```python
from build123d import *

# Parameters (mm, degrees)
BASE_EXTRUDE_DEPTH = 5.55625
SKETCH4_R          = 3.175
I_D_DEPTH          = 6.55625
SKETCH5_OUTSIDE_W  = 106.392
SKETCH5_OUTSIDE_H  = 104.672
SKETCH5_OUTSIDE_R  = 5.55625
CUT_EXTRUDE3_DEPTH = 25.4
CUT_EXTRUDE3_TAPER = 60
SKETCH6_OUTSIDE_W  = 53.046
SKETCH6_OUTSIDE_H  = 51.326
SKETCH6_OUTSIDE_R  = 5.55625
CUT_EXTRUDE4_DEPTH = 10
CUT_EXTRUDE4_TAPER = 60


with BuildPart() as part:
    # Sketch2 → Base-Extrude (new body)
    with BuildSketch(Plane.XY):
        Polygon((3.207902433, -5.55625), (6.415804866, 0), (3.207902433, 5.55625), (-3.207902433, 5.55625), (-6.415804866, 0), (-3.207902433, -5.55625), align=None)
    extrude(amount=-BASE_EXTRUDE_DEPTH)

    # Sketch4 → I.D. (cut, through all)
    with BuildSketch(Plane.XY):
        Circle(SKETCH4_R)
    extrude(amount=-I_D_DEPTH, mode=Mode.SUBTRACT)

    # Sketch5 outside → Cut-Extrude3 (cut)
    with BuildSketch(Plane(origin=(0, 0, -5.55625), x_dir=(-1, 0, 0), z_dir=(0, 0, -1))):
        Rectangle(SKETCH5_OUTSIDE_W, SKETCH5_OUTSIDE_H)
        Circle(SKETCH5_OUTSIDE_R, mode=Mode.SUBTRACT)
    extrude(amount=-CUT_EXTRUDE3_DEPTH, taper=CUT_EXTRUDE3_TAPER, mode=Mode.SUBTRACT)

    # Sketch6 outside → Cut-Extrude4 (cut)
    with BuildSketch(Plane.XY):
        Rectangle(SKETCH6_OUTSIDE_W, SKETCH6_OUTSIDE_H)
        Circle(SKETCH6_OUTSIDE_R, mode=Mode.SUBTRACT)
    extrude(amount=-CUT_EXTRUDE4_DEPTH, taper=CUT_EXTRUDE4_TAPER, mode=Mode.SUBTRACT)


solid = part.part
```
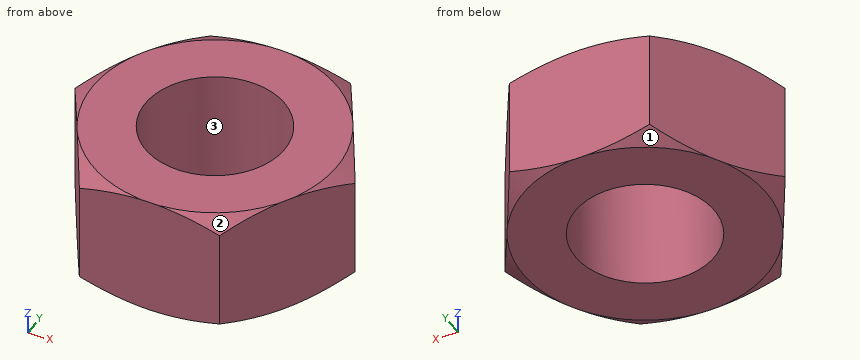
Geometry: final body of the model. Coordinates: model frame, mm. Face numbers are marked on the shaded views. Coordinates: 2 decimals unless noted, no trailing zeros. Loops run counter-clockwise (first coordinate to the right, second up) from the corner with the lowest first, then second, coordinate; pieces in that order, holes last. Notation, with made-up numbers: (-4, 69.5) -> (33, 69.5) arc R33 ccw to (33, 98.5) -> close; hole circle Ø10 at (28.25, -33). An arc over 180 degrees is marked (long way). Use a Markdown table: item, result. Add a question column.
(1) Line query: line 1 along Y through (x, z) = (0, -4.3) (3 decimals); line 2 along X through (y, z) = (-1.75, -2.55); line 3 along Y through (x, z) = (2.5, -4.2). Output: solid intervals per line, ascending.
(2) Mould query, pull axis X, two halves, no side actions, for the marked faces 1, 2 and 3. Classes: pulls with the +X half, pulls with the -X half, needs draft (parallel to the pull), parting line crosses it, or undercut.
(3) Section query A-A, the plane z = -1.45. Return loops of the section in (x, y) (3 decimals), plus the area to 3 significant figures.
(4) Pin query (flat end, axial travel): pin 1 Ø1.5 at (y, z) = (-1, -5) entering from +X; pin 2 Ø5.5 at (x, y) = (0, 0) entering from +Z. Return the tip coordinate at first contact, or that it passes through.
Answer:
| question | item | result |
|---|---|---|
| 1 | line 1 | y = -5.556 to -3.175, 3.175 to 5.556 |
| 1 | line 2 | x = -5.41 to -2.65, 2.65 to 5.41 |
| 1 | line 3 | y = -5.56 to -1.96, 1.96 to 5.56 |
| 2 | face 1 | pulls with the -X half |
| 2 | face 2 | pulls with the +X half |
| 2 | face 3 | undercut |
| 3 | outline | (-6.416, 0) -> (-3.208, -5.556) -> (3.208, -5.556) -> (6.416, 0) -> (3.208, 5.556) -> (-3.208, 5.556) -> close; hole circle Ø6.35 at (0, 0) |
| 3 | area | 75.3 mm^2 |
| 4 | pin 1 | stops at x = 6.27 |
| 4 | pin 2 | passes through |
